```python
from build123d import *

# Parameters (mm, degrees)
SKETCH1_W           = 50
SKETCH1_H           = 10
BOSS_EXTRUDE1_DEPTH = 90
SKETCH2_W           = 50
SKETCH2_H           = 20
BOSS_EXTRUDE2_DEPTH = 30
SKETCH3_R           = 15.0006
CUT_EXTRUDE1_DEPTH  = 108.238052948


with BuildPart() as part:
    # Sketch1 → Boss-Extrude1 (new body)
    with BuildSketch(Plane.XY):
        with Locations((25, -5)):
            Rectangle(SKETCH1_W, SKETCH1_H)
    extrude(amount=BOSS_EXTRUDE1_DEPTH)

    # Sketch2 → Boss-Extrude2 (add)
    with BuildSketch(Plane(origin=(0, 0, 0), x_dir=(1, 0, 0), z_dir=(0, 1, 0))):
        with Locations((25, -10)):
            Rectangle(SKETCH2_W, SKETCH2_H)
    extrude(amount=BOSS_EXTRUDE2_DEPTH)

    # Sketch3 → Cut-Extrude1 (cut, through all)
    with BuildSketch(Plane(origin=(0, 0, 0), x_dir=(1, 0, 0), z_dir=(0, 1, 0))):
        with Locations(Location((25.294928994, -50, 0), (0, 0, 270))):
            Circle(SKETCH3_R)
    extrude(amount=-CUT_EXTRUDE1_DEPTH, mode=Mode.SUBTRACT)


solid = part.part
```
Geometry: final body of the model. Coordinates: model frame, mm. A direction names the side the tool comes from. Coordinates: 2 decimals unless noted, no trailing zeros. Order: outer loops, then holes, each group sorted by start corner. A loop starts at its lowest first (then second) coordinate and runs counter-clockwise, first axis right, second up. Notation, with made-up numbers: (45.25, -26.5) -> (73.25, -26.5) arc R4 ccw to (73.25, -21.5) -> close; hole circle Ø4 at (-13.75, 43). An arc over 180 degrees is marked (long way). Write each question's results on one line, items separated by ' | '. Start each with the question number.
1) First-contact query: pin 1 (6 mm diameter, centred on x = 13, z = 35.5, fed in from +Y); pin 2 (15 mm diameter, centred on x = 35, y = 11.5, fed in from +Z); pin 3 (18 mm diameter, centred on x = 25.29, z = 50, fed in from +Y). Flat tips, straight axial feed; report the tip coordinate or a pass-through.
2) Cut plane D-D, the plane x = 7.5. Output: boundary loops of the cut face in (y, z), and give its area (3 significant figures).
3) Cut plane A-A, the plane x = 36. Output: boundary loops of the cut face in (y, z), and give its area (3 significant figures).
4) Mould query, pull axis X, two halves, no side actions, for faces 3 (the flat face through (50, -4, 26)), 4 (the flat face through (0, -4, 26)), 5 (the flat face through (25, 10, 0)), 6 (the cylindrical face through (19.55, -4.93, 63.857)). Classes: released by +X, released by -X, zero draft, split by the parting line, or undercut.
5) Material intervals for line 1 along X through (y, z) = (-4, 50); line 2 along Z through (x, y) = (9, 28.5); line 3 along Y through (x, z) = (6, 20.5), sorted ascending.
6) Set-up query: faces 1 (the flat face through (25, -5, 90)), 2 (the flat face through (25, 15, 20)). Return all of +Z, -Z, +X, -X, +Y, -Y with unobstructed straight access to the full face (end or side cutting, diameter ignored); none if empty.
7) Cut plane B-B, the plane z = 50. Output: boundary loops of the cut face in (x, y), and give its area (3 significant figures).
8) Cut plane C-C, the plane y = -5. Output: boundary loops of the cut face in (x, z), and give its area (3 significant figures).
Checks:
1) pin 1: y = 0 | pin 2: z = 20 | pin 3: through
2) outline: (-10, 0) -> (30, 0) -> (30, 20) -> (0, 20) -> (0, 90) -> (-10, 90) -> close | area: 1,500 mm^2
3) outline: (-10, 0) -> (30, 0) -> (30, 20) -> (0, 20) -> (0, 39.49) -> (-10, 39.49) -> close; (-10, 60.51) -> (0, 60.51) -> (0, 90) -> (-10, 90) -> close | area: 1,290 mm^2
4) face 3: released by +X | face 4: released by -X | face 5: zero draft | face 6: undercut
5) line 1: 0 to 10.29, 40.3 to 50 | line 2: 0 to 20 | line 3: -10 to 0
6) face 1: +Z, +X, -X, +Y, -Y | face 2: +Z, +X, -X, +Y
7) outline: (0, -10) -> (10.29, -10) -> (10.29, 0) -> (0, 0) -> close; (40.3, -10) -> (50, -10) -> (50, 0) -> (40.3, 0) -> close | area: 200 mm^2
8) outline: (0, 0) -> (50, 0) -> (50, 90) -> (0, 90) -> close; hole circle Ø30 at (25.29, 50) | area: 3,790 mm^2
